```python
from build123d import *

# Parameters (mm, degrees)
BOSS_EXTRUDE1_DEPTH      = 355.6
BOSS_EXTRUDE1_DEPTH_BACK = 355.6
SKETCH1_W                = 25.4
SKETCH1_H                = 25.4
SKETCH1_W_2              = 19.05
SKETCH1_H_2              = 19.05
SKETCH2_R                = 6.35
CUT_EXTRUDE1_DEPTH       = 495.648289191


with BuildPart() as part:
    # Sketch1 → Boss-Extrude1 (new, two sides: drawn at the far end of the back side and taken through both)
    with BuildSketch(Plane.XY.offset(-BOSS_EXTRUDE1_DEPTH_BACK)):
        with Locations((330.2, 79.375)):
            Rectangle(SKETCH1_W, SKETCH1_H)
        with Locations((330.2, 79.375)):
            Rectangle(SKETCH1_W_2, SKETCH1_H_2, mode=Mode.SUBTRACT)
    extrude(amount=BOSS_EXTRUDE1_DEPTH + BOSS_EXTRUDE1_DEPTH_BACK)

    # Sketch2 → Cut-Extrude1 (cut, through all)
    with BuildSketch(Plane(origin=(0, 92.075, 0), x_dir=(1, 0, 0), z_dir=(0, 1, 0))):
        with Locations(Location((330.2, -330.2, 0), (0, 0, 270))):
            Circle(SKETCH2_R)
        with Locations(Location((330.2, 330.2, 0), (0, 0, 270))):
            Circle(SKETCH2_R)
    extrude(amount=-CUT_EXTRUDE1_DEPTH, mode=Mode.SUBTRACT)


solid = part.part
```
Work out the finished part from the listing and answer in its coordinate system (mm). A direction names the side the tool comes from. Give positions to 0.01 mm unless a question says otherwise; leave off trailing zeros. Loops run counter-clockwise (first coordinate to the right, second up) from the corner with the lowest first, then second, coordinate; pieces in that order, holes last. Notation, with made-up numbers: (66, 59.25) - (88, 59.25) arc R26 cw to (88, 92.25) - close; hole circle Ø1 at (77.25, 79). An arc over 180 degrees is marked (long way). Use CSV: the item, a comma, the result in double quotes. Start each with the question number.
(1) A tool of negligible diameter and unlimited length cuts with its end or side. For faces 4 (the face through (330, 69.85, -5)), 5 (the face through (324.566, 90.51, -327.27)), from which of +Z, -Z, +X, -X, +Y, -Y can it reach the whole face along a straight path? Write none if from no direction.
(2) Find section A-A, the plane z = -330.2. Determine the outline of the cut face in (x, y) (3 decimals), plus the area to 3 significant figures.
(3) Find section C-C, the plane x = 330.2. Determine the outline of the cut face in (y, z) (3 decimals).
(4) Determine the mould class of faces 1 (the face through (341, 80, 355.6)), 2 (the face through (339.725, 79, -5)), 3 (the face through (317.5, 79, -5)) for opening direction X: released by +X, released by -X, zero draft, split by the parting line, or undercut.
(5) Find section D-D, the plane y = 83.5. Determine the outline of the cut face in (x, z) (3 decimals), plus the area to 3 significant figures.
(6) Find the intervals of material crossed by L1, parallel to Z at x = 330.2, y = 68.5; L2, parallel to X at y = 72.5, z = -313.5 (3 decimals); L3, parallel to Y at x = 327.5, z = -149 (3 decimals), in increasing order.
(7) Find section B-B, the plane z = -146. Determine the outline of the cut face in (x, y) (3 decimals), plus the area to 3 significant figures.
Results found:
1,face 4,"+Z, -Z"
1,face 5,"+Y, -Y"
2,outline,"(317.5, 66.675) - (323.85, 66.675) - (323.85, 69.85) - (320.675, 69.85) - (320.675, 88.9) - (323.85, 88.9) - (323.85, 92.075) - (317.5, 92.075) - close; (336.55, 66.675) - (342.9, 66.675) - (342.9, 92.075) - (336.55, 92.075) - (336.55, 88.9) - (339.725, 88.9) - (339.725, 69.85) - (336.55, 69.85) - close"
2,area,"202 mm^2"
3,outline,"(66.675, -355.6) - (69.85, -355.6) - (69.85, -336.55) - (66.675, -336.55) - close; (66.675, -323.85) - (69.85, -323.85) - (69.85, 323.85) - (66.675, 323.85) - close; (66.675, 336.55) - (69.85, 336.55) - (69.85, 355.6) - (66.675, 355.6) - close; (88.9, -355.6) - (92.075, -355.6) - (92.075, -336.55) - (88.9, -336.55) - close; (88.9, -323.85) - (92.075, -323.85) - (92.075, 323.85) - (88.9, 323.85) - close; (88.9, 336.55) - (92.075, 336.55) - (92.075, 355.6) - (88.9, 355.6) - close"
4,face 1,"zero draft"
4,face 2,"undercut"
4,face 3,"released by -X"
5,outline,"(317.5, -355.6) - (320.675, -355.6) - (320.675, 355.6) - (317.5, 355.6) - close; (339.725, -355.6) - (342.9, -355.6) - (342.9, 355.6) - (339.725, 355.6) - close"
5,area,"4,520 mm^2"
6,L1,"-355.6 to -336.55, -323.85 to 323.85, 336.55 to 355.6"
6,L2,"317.5 to 320.675, 339.725 to 342.9"
6,L3,"66.675 to 69.85, 88.9 to 92.075"
7,outline,"(317.5, 66.675) - (342.9, 66.675) - (342.9, 92.075) - (317.5, 92.075) - close; hole (320.675, 69.85) - (339.725, 69.85) - (339.725, 88.9) - (320.675, 88.9) - close"
7,area,"282 mm^2"
